Source: CAD feature listing. Evaluate the final solid. Frame: model axes, mm. A direction names the side the tool comes from. Coordinates: 2 decimals unless noted, no trailing zeros. Loops run counter-clockwise (first coordinate to the right, second up) from the corner with the lowest first, then second, coordinate; pieces in that order, holes last.
Item 1: Section query B-B, the plane y = -91.5. Return the cut outline in (x, z).
Item 2: Pin query (flat end, axial travel): pin 1 Ø3 at (x, z) = (33.5, -2.5) entering from -Y; pin 2 Ø1 at (y, z) = (-66.5, -2) entering from -X; pin 3 Ø4 at (x, z) = (32.5, 1.5) entering from +Y. Return the tip coordinate at first contact, or that it passes through.
Item 3: Section query C-C, the plane y = -52. Return the cut outline in (x, z), then the cut area to 3 significant figures.
Item 4: Pull-direction query (X, two-part tool) for faces 4 (the flat face through (91.5, -88.9, 0.9)), 5 (the cylindrical face through (32.19, -0.33, 2.52)), 6 (the flat face through (84.049, -98, 0)); classes: +X half, -X half, draft (parallel to the pull), parting line (faces both ways), or undercut.
Item 5: Line query: probe 1 along X at (y, z) = (-93.5, 3); probe 2 along X at (y, z) = (-39.5, 0.25); probe 3 along Y at (x, z) = (-10, 0). Output: solid intervals per line, ascending.
Item 6: Reachability of faces 1 (the flat face through (-13, -5.08, 0)), 2 (the cylindrical face through (86.362, -57.594, 0.112)), 3 (the flat face through (89, -103, 3.81)) from +Z, -Z, +X, -X, +Y, -Y: full face, straight path, thin tool, end or side. Return the list, or none.
Item 7: Section query A-A, the plane x = -3. Return the cut outline in (y, z).
Item 8: Section query D-D, the plane x = 30. Return the cut outline in (y, z).
```python
from build123d import *

# Parameters (mm, degrees)
F0_R      = 2.54
F3_W      = 25.3560190095
F3_H      = 10.16
F4_DEPTH  = 3.81
F6_DEPTH  = 7.62
F7_R      = 1.27
F9_DEPTH  = 25.4
F11_DEPTH = 3.81
F12_R     = 1.27
F14_DEPTH = 25.4


with BuildPart() as f2:
    # F2: sweep along a path in F1
    with BuildLine(Plane.XY) as f2_path:
        Line((0, 0), (63.5, 0))
        ThreePointArc((63.5, 0), (81.4605122421, -7.4394877579), (88.9, -25.4))
        Line((88.9, -25.4), (88.9, -88.9))
    # F0 (on Right) → F2 (sweep)
    with BuildSketch(Plane.YZ):
        Circle(F0_R)
    sweep(path=f2_path.line)

    # F3 (on Top) → F4 (join, symmetric)
    with BuildSketch(Plane.XY):
        with Locations((-12.6780095048, 0)):
            Rectangle(F3_W, F3_H)
    extrude(amount=F4_DEPTH, both=True)

    # F5 (on face) → F6 (join, through all)
    with BuildSketch(Plane.XY.offset(3.81)):
        Polygon((-25.3560190095, -5.08), (-25.3560190095, 5.08), (-49.4670197368, 0), align=None)
    extrude(amount=-F6_DEPTH)

    # F7
    f7_edges = [f2.edges().sort_by_distance(p)[0] for p in [
        (-49.46702, 0, 0),
    ]]
    fillet(f7_edges, radius=F7_R)

    # F8 (on face) → F9 (cut)
    with BuildSketch(Plane.XZ.offset(5.08)):
        Polygon((-46.2558194995, -3.1080117915), (-37.216514349, 0), (-46.2558194995, 3.528587753), align=None)
    extrude(amount=-F9_DEPTH, mode=Mode.SUBTRACT)

    # F10 (on Top) → F11 (join, symmetric)
    with BuildSketch(Plane.XY):
        Polygon((94.2088630664, -88.9), (84.0488630664, -88.9), (84.0488630664, -107.95), (89.1288630664, -128.7725716829), (94.2088630664, -107.95), align=None)
    extrude(amount=F11_DEPTH, both=True)

    # F12
    f12_edges = [f2.edges().sort_by_distance(p)[0] for p in [
        (89.128863, -128.772572, 0),
    ]]
    fillet(f12_edges, radius=F12_R)

    # F13 (on face) → F14 (cut)
    with BuildSketch(Plane.YZ.offset(94.2088630664)):
        Polygon((-128.7030428648, -2.9382649809), (-114.0688881278, 0), (-128.7030428648, 3.176004393), align=None)
    extrude(amount=-F14_DEPTH, mode=Mode.SUBTRACT)


solid = f2.part
```
Verdict:
1. outline: (84.05, -3.81) - (94.21, -3.81) - (94.21, 3.81) - (84.05, 3.81) - close
2. pin 1: stops at y = -2.33
2. pin 2: stops at x = 86.85
2. pin 3: stops at y = 2.54
3. outline: circle Ø5.08 at (88.9, 0)
3. area: 20.3 mm2
4. face 4: draft
4. face 5: undercut
4. face 6: -X half
5. probe 1: x = 84.05 to 94.21
5. probe 2: x = 86.37 to 91.43
5. probe 3: y = -5.08 to 5.08
6. face 1: +Z, -Z, -X, -Y
6. face 2: none
6. face 3: +Z, +X, -X, +Y, -Y
7. outline: (-5.08, -3.81) - (5.08, -3.81) - (5.08, 3.81) - (-5.08, 3.81) - close
8. outline: circle Ø5.08 at (0, 0)
